from build123d import *

# Parameters (mm, degrees)
SKETCH1_W           = 50.8
SKETCH1_H           = 66.2
SKETCH1_R           = 2
SKETCH1_R_2         = 7
BOSS_EXTRUDE1_DEPTH = 10
SKETCH2_W           = 50.8
SKETCH2_H           = 50.8
BOSS_EXTRUDE2_DEPTH = 10
FILLET2_R           = 20
SKETCH3_R           = 1.25
CUT_EXTRUDE1_DEPTH  = 105.726882891
SKETCH4_R           = 1.25
SKETCH4_R_2         = 1.5
CUT_EXTRUDE2_DEPTH  = 105.726882939
CUT_EXTRUDE3_DEPTH  = 105.726882939
FILLET3_DEPTH       = 10.364318194
FILLET3_START       = -1
FILLET3_2_DEPTH     = 53


with BuildPart() as part:
    # Sketch1 → Boss-Extrude1 (new body)
    with BuildSketch(Plane(origin=(0, 0, 0), x_dir=(1, 0, 0), z_dir=(0, 1, 0))):
        with Locations((25.4, 33.1)):
            Rectangle(SKETCH1_W, SKETCH1_H)
        with Locations(Location((14.086291501, 20, 0), (0, 0, 270))):
            Circle(SKETCH1_R, mode=Mode.SUBTRACT)
        with Locations(Location((25.4, 8.686291501, 0), (0, 0, 270))):
            Circle(SKETCH1_R, mode=Mode.SUBTRACT)
        with Locations(Location((36.713708499, 20, 0), (0, 0, 270))):
            Circle(SKETCH1_R, mode=Mode.SUBTRACT)
        with Locations(Location((25.4, 31.313708499, 0), (0, 0, 270))):
            Circle(SKETCH1_R, mode=Mode.SUBTRACT)
        with Locations(Location((25.4, 20, 0), (0, 0, 270))):
            Circle(SKETCH1_R_2, mode=Mode.SUBTRACT)
    extrude(amount=BOSS_EXTRUDE1_DEPTH)

    # Sketch2 → Boss-Extrude2 (add)
    with BuildSketch(Plane(origin=(0, 0, -66.2), x_dir=(-1, 0, 0), z_dir=(0, 0, -1))):
        with Locations((-25.4, 25.4)):
            Rectangle(SKETCH2_W, SKETCH2_H)
    extrude(amount=BOSS_EXTRUDE2_DEPTH)

    # Fillet2
    fillet2_edges = [part.edges().sort_by_distance(p)[0] for p in [
        (25.4, 10, -66.2),
    ]]
    fillet(fillet2_edges, radius=FILLET2_R)

    # Sketch3 → Cut-Extrude1 (cut, through all)
    with BuildSketch(Plane(origin=(50.8, 0, 0), x_dir=(0, 0, -1), z_dir=(1, 0, 0))):
        with Locations((61.2, 5)):
            Circle(SKETCH3_R)
        with Locations((31.2, 5)):
            Circle(SKETCH3_R)
        with Locations((5, 5)):
            Circle(SKETCH3_R)
    extrude(amount=-CUT_EXTRUDE1_DEPTH, mode=Mode.SUBTRACT)

    # Sketch4 → Cut-Extrude2 (cut, through all)
    with BuildSketch(Plane(origin=(50.8, 0, 0), x_dir=(0, 0, -1), z_dir=(1, 0, 0))):
        with Locations((71.2, -9.2)):
            Circle(SKETCH4_R)
        with Locations((71.2, 30.8)):
            Circle(SKETCH4_R)
        with Locations((71.2, 10.8)):
            Circle(SKETCH4_R_2)
        with Locations((71.2, 40.8)):
            Circle(SKETCH4_R_2)
    extrude(amount=-CUT_EXTRUDE2_DEPTH, mode=Mode.SUBTRACT)

    # Sketch5 → Cut-Extrude3 (cut, through all)
    with BuildSketch(Plane(origin=(0, 0, 0), x_dir=(-1, 0, 0), z_dir=(0, -1, 0))):
        with BuildLine():
            ThreePointArc((-25.4, 4), (-36.713708499, 8.686291501), (-41.4, 20))
            Line((-41.4, 20), (-41.4, 50))
            Line((-41.4, 50), (-50.8, 50))
            Line((-50.8, 50), (-50.8, 0))
            Line((-50.8, 0), (0, 0))
            Line((0, 0), (0, 50))
            Line((0, 50), (-9.4, 50))
            Line((-9.4, 50), (-9.4, 20))
            ThreePointArc((-9.4, 20), (-14.086291501, 8.686291501), (-25.4, 4))
        make_face()
    extrude(amount=-CUT_EXTRUDE3_DEPTH, mode=Mode.SUBTRACT)

    # Fillet3: read off the stored shape, not the designer's step
    # Fillet3 outline → Fillet3 (add)
    with BuildSketch(Plane(origin=(0, 0, 0), x_dir=(1, 0, 0), z_dir=(0, 1, 0))):
        with BuildLine():
            ThreePointArc((0, 50), (6.680109889, 46.87367083), (9.4, 40.018016229))
            Line((9.4, 40.018016229), (9.4, 50))
            Line((9.4, 50), (0, 50))
        make_face()
        with BuildLine():
            ThreePointArc((41.4, 40.018016229), (44.119890111, 46.87367083), (50.8, 50))
            Line((50.8, 50), (41.4, 50))
            Line((41.4, 50), (41.4, 40.018016229))
        make_face()
    extrude(amount=FILLET3_DEPTH)

    # Fillet3 2 outline → Fillet3 2 (cut)
    with BuildSketch(Plane.YZ.offset(FILLET3_START)):
        with BuildLine():
            ThreePointArc((10, -46.2), (10.091287885, -48.108712115), (10.364318194, -50))
            ThreePointArc((10.364318194, -50), (10.586120766, -51.006380458), (10.859467092, -52))
            Line((10.859467092, -52), (12, -52))
            Line((12, -52), (12, -39))
            Line((12, -39), (10, -39))
            Line((10, -39), (10, -46.2))
        make_face()
    extrude(amount=FILLET3_2_DEPTH, mode=Mode.SUBTRACT)


solid = part.part
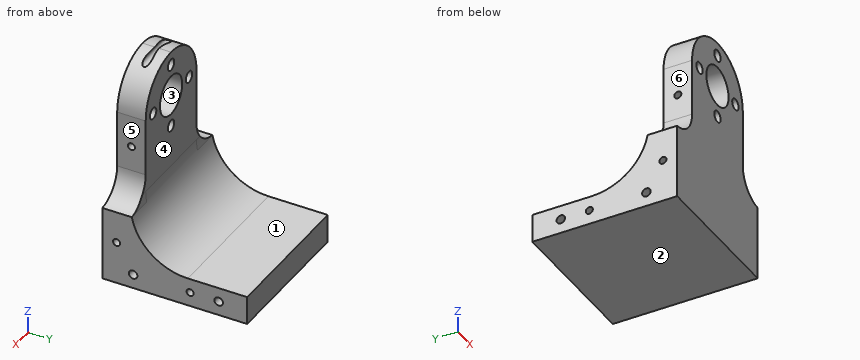
Verification items for the finished model (mm, model axes). Face numbers are marked on the shaded views. A direction names the side the tool comes from. Coordinates: 2 decimals unless noted, no trailing zeros. Loops run counter-clockwise (first coordinate to the right, second up) from the corner with the lowest first, then second, coordinate; pieces in that order, holes last. Notation, with made-up numbers: M -16,66.5 L 3,66.5 A25 ccw 3,97.5 Z; hole C -23,72.5 d8. An arc over 180 degrees is marked long. One line per item, written item: value.
1. Set-up check for the marked faces 4, 5 and 6: record each of +Z, -Z, +X, -X, +Y, -Y from which the full face is reachable in a straight line by a thin tool's end or side.
Answers follow:
face 4: +Z, +X, -X, +Y
face 5: +Z, +X, +Y, -Y
face 6: +Z, -X, +Y, -Y
2. Material ranges on line 1 along X through (y, z) = (4.25, -20); line 2 along Y through (x, z) = (31, -71.2); line 3 along Z through (x, y) = (26, 31), recorded low to high. Write a range as from..to.
Answers follow:
line 1: 9.4..12.09, 16.09..18.4, 32.4..34.71, 38.71..41.4
line 2: 0..9.3, 12.3..29.55, 32.05..39.3, 42.3..50.8
line 3: -76.2..-72.43, -69.97..-66.2
3. Section check C-C on z = -61.2. Record the cut outline in (x, y), plus the area to 3 significant figures.
Answers follow:
outline: M 0,0 L 50.8,0 L 50.8,3.75 L 0,3.75 Z; M 0,6.25 L 50.8,6.25 L 50.8,16.77 L 0,16.77 Z
area: 725 mm^2
4. Section check A-A on z = -71.2. Record the cut outline in (x, y), plus the area to 3 significant figures.
Answers follow:
outline: M 0,0 L 50.8,0 L 50.8,9.3 L 0,9.3 Z; M 0,12.3 L 50.8,12.3 L 50.8,29.55 L 0,29.55 Z; M 0,32.05 L 50.8,32.05 L 50.8,39.3 L 0,39.3 Z; M 0,42.3 L 50.8,42.3 L 50.8,50.8 L 0,50.8 Z
area: 2,150 mm^2
5. Section check B-B on y = 40.8. Record the cut outline in (x, z), plus the area to 3 significant figures.
Answers follow:
outline: M 0,-76.2 L 50.8,-76.2 L 50.8,-72.7 L 0,-72.7 Z; M 0,-69.7 L 50.8,-69.7 L 50.8,-66.2 L 0,-66.2 Z
area: 356 mm^2
6. Gauge pin test, flat ends, axial feed: P1, Ø3, axis at y = 5, z = -31.2, coming from the +X side; P2, Ø5, axis at x = 31.5, z = -58.5, coming from the -Y side; P3, Ø2.5, axis at y = 40.8, z = -71.2, coming from the +X side; P4, Ø1.5, axis at x = 37, y = 29.5, coming from the +Z side. Record the tip position at first contact, or that the pin passes through.
Answers follow:
P1: x = 41.4
P2: y = 0
P3: through
P4: z = -66.16
7. Mould release check, pull along Z, two halves, no side actions. Record for the marked faces 1, 2 and 3: pulls with the +Z half, pulls with the -Z half, needs draft (parallel to the pull), parting line crosses it, or undercut.
Answers follow:
face 1: pulls with the +Z half
face 2: pulls with the -Z half
face 3: undercut
8. Section check D-D on x = 4. Record the cut outline in (y, z).
Answers follow:
outline: M 0,-76.2 L 50.8,-76.2 L 50.8,-66.2 L 30,-66.2 A20 cw 10.18,-48.9 L 0,-48.9 Z; hole C 5,-61.2 d2.5; hole C 10.8,-71.2 d3; hole C 30.8,-71.2 d2.5; hole C 40.8,-71.2 d3
